Autodesk Inventor part; units mm, degrees
ref_plane "Work Plane1" through (6.35, 0, 177.8) normal (0, 1, 0) x (1, 0, 0)
ref_plane "YZ Plane" through (0, 0, 0) normal (1, 0, 0) x (0, 1, 0)
ref_plane "XZ Plane" through (0, 0, 0) normal (0, 1, 0) x (-1, 0, 0)
sketch "Sketch1" plane through (0, 0, 0) normal (1, 0, 0) x (0, 1, 0)
  arc A0 (165.1, 0) -> (-165.1, 0) centre (0, 0) ccw
  arc A1 (114.3, 0) -> (-114.3, 0) centre (0, 0) ccw
  line L0 (165.1, 0) -> (114.3, 0)
  line L1 (-114.3, 0) -> (-165.1, 0)
  circle A2 centre (0, 0) radius 130.81 construction
  circle A3 centre (0, 0) radius 147.32 construction
  line L2 (0, 0) -> (167.0124, 167.0124) construction
  line L3 (0, 0) -> (-143.9917, 143.9917) construction
  line L4 (0, 0) -> (0, 334.0248) construction
  point P0 (146.7716, 12.7)
  point P1 (142.4086, 37.7225)
  point P2 (130.192, 12.7)
  point P3 (125.2833, 37.6212)
  point P4 (133.8122, 61.6236)
  point P5 (115.6509, 61.1239)
  point P6 (12.7, 146.7716)
  point P7 (37.7225, 142.4086)
  point P8 (12.7, 130.192)
  point P9 (37.6212, 125.2833)
  point P10 (61.6236, 133.8122)
  point P11 (61.1239, 115.6509)
  point P12 (-146.7716, 12.7)
  point P13 (-142.4086, 37.7225)
  point P14 (-130.192, 12.7)
  point P15 (-125.2833, 37.6212)
  point P16 (-133.8122, 61.6236)
  point P17 (-115.6509, 61.1239)
  point P18 (-61.6236, 133.8122)
  point P19 (-37.7225, 142.4086)
  point P20 (-12.7, 146.7716)
  point P21 (-12.7, 130.192)
  point P22 (-37.6212, 125.2833)
  point P23 (-61.1239, 115.6509)
  dimension "d1" = 228.6
  dimension "d2" = 50.8
  dimension "d3" = 261.62
  dimension "d4" = 330.2
  dimension "d5" = 294.64
  dimension "d6" = 25.4
  dimension "d7" = 25.4
  dimension "d8" = 12.7
  dimension "d9" = 12.7
  dimension "d10" = 25.4
  dimension "d11" = 25.4
  dimension "d12" = 45
  dimension "d13" = 45
extrude "Extrusion1" add sketch "Sketch1" along normal blind 6.35
hole "Hole1" at (0, 146.7716, 12.7) at (0, 142.4086, 37.7225) at (0, 130.192, 12.7) at (0, 125.2833, 37.6212) at (0, 133.8122, 61.6236) at (0, 115.6509, 61.1239) at (0, 61.6236, 133.8122) at (0, 37.7225, 142.4086) at (0, 12.7, 146.7716) at (0, 12.7, 130.192) at (0, 37.6212, 125.2833) at (0, 61.1239, 115.6509) at (0, -61.6236, 133.8122) at (0, -61.1239, 115.6509) at (0, -37.7225, 142.4086) at (0, -37.6212, 125.2833) at (0, -12.7, 146.7716) at (0, -12.7, 130.192) at (0, -115.6509, 61.1239) at (0, -133.8122, 61.6236) at (0, -142.4086, 37.7225) at (0, -125.2833, 37.6212) at (0, -146.7716, 12.7) at (0, -130.192, 12.7) direction (1, 0, 0) diameter 6.604 end through all
sketch "Sketch2" plane through (6.35, 0, 0) normal (1, 0, 0) x (0, 0, -1)
  circle A0 centre (-121.4655, -96.1901) radius 3.302
  point P0 (0, 0)
extrude "Extrusion2" cut sketch "Sketch2" against normal blind 25.4
ref_plane "Work Plane1" through (6.35, 0, 177.8) normal (0, 1, 0) x (1, 0, 0)
mirror "Mirror1" about plane through (6.35, 0, 177.8) normal (0, 1, 0) of "Extrusion2"
properties part number "13in inner coil" material "Copper"
Could you check a few things on this model? Use its own coordinates, in mm. Give positions to 0.01 mm unless a question says otherwise; leave off trailing zeros. Order: outer loops, then holes, each group sorted by start corner. A loop starts at its lowest first (then second) coordinate and runs counter-clockwise, first axis right, second up. Notation, with made-up numbers: (-10, 64) - (29, 64) arc R9 ccw to (29, 78) - close; hole circle Ø3 at (59.25, 74.5). An arc over 180 degrees is marked (long way). One line per item, written item: value. Start each with the question number.
1. Imagine slicing it at D-D on x = 2.25. Give the number of separate pieces and of enclosed holes in the cut face, plus the area to 3 significant figures.
2. If I drill on probe 1 along Z at (x, y) = (4.5, -12); probe 2 along Y at (x, z) = (2.25, 12.7); probe 3 along Y at (x, z) = (2, 60.5), over which ranges is the centre line in solid material (lowest first)?
3. Thinking about a two-plate mould opening in Z: for faces 1 (the face through (3.131, -2.513, 114.272)), 2 (the face through (0, -2, 120)), 3 (the face through (3.219, -128.557, 37.191)), which applies, +Z half, -Z half, draft (parallel to the pull), parting line (faces both ways), or undercut?
4. Imagine slicing it at B-B on z = 12.7. List the corners of the cut face in (x, y) for me, plus the area to 3 significant figures.
5. Imagine slicing it at C-C on y = 12.7. List the corners of the cut face in (x, z) for me, plus the area to 3 significant figures.
6. Imagine slicing it at A-A on z = 70. List the corners of the cut face in (x, y) for me.
7. For P1, Ø8.5, axis at y = -115.65, z = 61.12, coming from the +X side; P2, Ø6, axis at y = -125.28, z = 37.62, coming from the -X side; P3, Ø1.5, axis at x = 2, z = 79.5, coming from the -Y side; P4, Ø3, axis at x = 1, z = 145.5, coming from the -Y side, each with a flat end and sliding along its axis, tell me the tip position at first contact or that it passes through.
Values:
1. separate pieces: 1
1. enclosed holes: 26
1. area: 21,400 mm²
2. probe 1: 113.67 to 126.97, 133.42 to 143.54, 150 to 164.66
2. probe 2: -164.61 to -150.07, -143.47 to -133.49, -126.89 to -113.59, 113.59 to 126.89, 133.49 to 143.47, 150.07 to 164.61
2. probe 3: -153.62 to -136.92, -130.71 to -118.89, -112.41 to -96.98, 96.98 to 112.41, 118.89 to 130.71, 136.92 to 153.62
3. face 1: -Z half
3. face 2: draft
3. face 3: undercut
4. outline: (0, -164.61) - (6.35, -164.61) - (6.35, -150.07) - (0, -150.07) - close; (0, -143.47) - (6.35, -143.47) - (6.35, -133.49) - (0, -133.49) - close; (0, -126.89) - (6.35, -126.89) - (6.35, -113.59) - (0, -113.59) - close; (0, 113.59) - (6.35, 113.59) - (6.35, 126.89) - (0, 126.89) - close; (0, 133.49) - (6.35, 133.49) - (6.35, 143.47) - (0, 143.47) - close; (0, 150.07) - (6.35, 150.07) - (6.35, 164.61) - (0, 164.61) - close
4. area: 480 mm²
5. outline: (0, 113.59) - (6.35, 113.59) - (6.35, 126.89) - (0, 126.89) - close; (0, 133.49) - (6.35, 133.49) - (6.35, 143.47) - (0, 143.47) - close; (0, 150.07) - (6.35, 150.07) - (6.35, 164.61) - (0, 164.61) - close
5. area: 240 mm²
6. outline: (0, -149.53) - (6.35, -149.53) - (6.35, -90.36) - (0, -90.36) - close; (0, 90.36) - (6.35, 90.36) - (6.35, 149.53) - (0, 149.53) - close
7. P1: x = 6.35
7. P2: through
7. P3: y = -145.11
7. P4: y = -80.76
